from build123d import *

# Parameters (mm, degrees)
SKETCH1_R           = 38
BOSS_EXTRUDE1_DEPTH = 5
FILLET1_R           = 4
SKETCH2_R           = 2
BOSS_EXTRUDE2_DEPTH = 2.3
SKETCH3_R           = 32.474473425
CUT_EXTRUDE1_DEPTH  = 2
SKETCH4_R           = 35.191697817
SKETCH4_R_2         = 32.740433986
CUT_EXTRUDE2_DEPTH  = 2
SKETCH5_R           = 31.128585578
BOSS_EXTRUDE3_DEPTH = 3


with BuildPart() as part:
    # Sketch1 → Boss-Extrude1 (new body)
    with BuildSketch(Plane(origin=(0, 0, 0), x_dir=(0, 0, -1), z_dir=(1, 0, 0))):
        Circle(SKETCH1_R)
    extrude(amount=BOSS_EXTRUDE1_DEPTH)

    # Fillet1
    fillet1_edges = [part.edges().sort_by_distance(p)[0] for p in [
        (5, 0, 38),
    ]]
    fillet(fillet1_edges, radius=FILLET1_R)

    # Sketch2 → Boss-Extrude2 (add)
    with BuildSketch(Plane.ZY):
        with Locations(Location((0, 0, 0), (0, 0, 180))):
            Circle(SKETCH2_R)
        with Locations(Location((0, 16.29, 0), (0, 0, 180))):
            Circle(SKETCH2_R)
        with Locations(Location((16.29, 0, 0), (0, 0, 180))):
            Circle(SKETCH2_R)
        with Locations(Location((-16.29, 0, 0), (0, 0, 180))):
            Circle(SKETCH2_R)
        with Locations(Location((0, -16.29, 0), (0, 0, 180))):
            Circle(SKETCH2_R)
    extrude(amount=BOSS_EXTRUDE2_DEPTH)

    # Sketch3 → Cut-Extrude1 (cut)
    with BuildSketch(Plane(origin=(5, 0, 0), x_dir=(0, 0, -1), z_dir=(1, 0, 0))):
        Circle(SKETCH3_R)
    extrude(amount=-CUT_EXTRUDE1_DEPTH, mode=Mode.SUBTRACT)

    # Sketch4 → Cut-Extrude2 (cut)
    with BuildSketch(Plane.ZY):
        Circle(SKETCH4_R)
        Circle(SKETCH4_R_2, mode=Mode.SUBTRACT)
    extrude(amount=-CUT_EXTRUDE2_DEPTH, mode=Mode.SUBTRACT)

    # Sketch5 → Boss-Extrude3 (add)
    with BuildSketch(Plane(origin=(3, 0, 0), x_dir=(0, 0, -1), z_dir=(1, 0, 0))):
        Circle(SKETCH5_R)
    extrude(amount=BOSS_EXTRUDE3_DEPTH)


solid = part.part
Verification items for the finished model (mm, model axes). A direction names the side the tool comes from. Coordinates: 2 decimals unless noted, no trailing zeros. Answer as a JSON object with one key per item and string values.
(1) Thickness scan on line 1 along Y through (x, z) = (1.2, 0) (3 decimals); line 2 along Y through (x, z) = (4, 0); line 3 along Z through (x, y) = (1.25, -28). Record the ranges inside material, lowest first.
Report:
{"line 1": "-37.995 to -35.192, -32.74 to 32.74, 35.192 to 37.995", "line 2": "-36.65 to -32.47, -31.13 to 31.13, 32.47 to 36.65", "line 3": "-25.68 to -21.32, -16.97 to 16.97, 21.32 to 25.68"}
(2) Gauge pin test, flat ends, axial feed: pin 1 Ø1.5 at (x, z) = (0, 7) entering from +Y; pin 2 Ø1 at (y, z) = (-28.5, -15.5) entering from -X; pin 3 Ø2 at (x, z) = (5, 7) entering from +Y. Record the tip position at first contact, or that the pin passes through.
Report:
{"pin 1": "y = 37.48", "pin 2": "x = 0", "pin 3": "y = 35.99"}
(3) Mould release check, pull along Z, two halves, no side actions. Record for faces 1 (the flat face through (5, -28, -17)), 2 (the cylindrical face through (-1.134, -18.273, 0.26)), 3 (the cylindrical face through (4.48, 9.35, -29.69)): pulls with the +Z half, pulls with the -Z half, needs draft (parallel to the pull), parting line crosses it, or undercut.
Report:
{"face 1": "needs draft", "face 2": "parting line crosses it", "face 3": "undercut"}
(4) Tool access check on faces 4 (the cylindrical face through (0.99, 9.83, 31.23)), 5 (the flat face through (-2.3, -16, 0)), 6 (the cylindrical face through (4.014, -31.702, 7.04)). Record the directions out of +Z, -Z, +X, -X, +Y, -Y that give a thin tool (end or side, any length) a straight path to the whole face; none if there is none.
Report:
{"face 4": "-X", "face 5": "+Z, -Z, -X, +Y, -Y", "face 6": "+X"}
